Model file for the job. Use its own axes, mm. Face numbers are marked on the shaded views. A direction names the side the tool comes from. Give positions to 0.01 mm unless a question says otherwise; leave off trailing zeros. Write each loop counter-clockwise with the first axis right and the second up, starting at its lowest first coordinate (ties: lowest second). Pieces come first, ordered by that corner, then holes. Notation, with made-up numbers: (55, 74.5) - (111, 74.5) arc R30 cw to (111, 108.5) - close; hole circle Ø5 at (53.25, -3). An arc over 180 degrees is marked (long way). One line per item, written item: value. Start each with the question number.
(1) Cut at C-C, the plane z = 10. List the corners of the cut face in (x, y), and give its area (3 significant figures).
(2) Mould opens along Y. For the marked faces 1, 2, 3 and 4 say: pulls with the +Y half, pulls with the -Y half, needs draft (parallel to the pull), parting line crosses it, or undercut.
(3) Probe L1, parallel to Y at x = -2.5, z = 8; L2, parallel to Y at x = -5, z = 7; L3, parallel to X at y = -4, z = 18. List the from-to ranges inside material, lowest first.
(4) Cut at A-A, the plane x = 1.75. List the corners of the cut face in (y, z).
(5) Drop flat-ended pins along their axis: P1, Ø6, axis at y = -1, z = 6.5, coming from the -X side; P2, Ø6, axis at x = 5.5, z = 12.5, coming from the +Y side; P3, Ø8, axis at y = 3.5, z = 6, coming from the -X side. Give the stop position or say it passes through.
(6) Cut at D-D, the plane y = -8.5. List the corners of the cut face in (x, z).
(7) Cut at B-B, the plane y = 3.75. List the corners of the cut face in (x, z).
(8) 3-axis set-ups, long thin cutter, end or side, ignore diameter. For the marked faces 5 and 6: which of +Z, -Z, +X, -X, +Y, -Y reach the whole face in a straight line?
Autodesk Inventor part; units mm, degrees
ref_plane "YZ Plane" through (0, 0, 0) normal (1, 0, 0) x (0, 1, 0)
ref_plane "XZ Plane" through (0, 0, 0) normal (0, 1, 0) x (-1, 0, 0)
ref_plane "XY Plane" through (0, 0, 0) normal (0, 0, 1) x (1, 0, 0)
sketch "Sketch1" plane through (0, 0, 0) normal (0, 0, 1) x (1, 0, 0)
  line L0 (-2.6795, 10) -> (7.3205, 7.3205)
  line L1 (7.3205, 7.3205) -> (10, -2.6795)
  line L2 (10, -2.6795) -> (2.6795, -10)
  line L3 (2.6795, -10) -> (-7.3205, -7.3205)
  line L4 (-7.3205, -7.3205) -> (-10, 2.6795)
  line L5 (-10, 2.6795) -> (-2.6795, 10)
  point P0 (0, 0)
  point P1 (0, 0)
  dimension "d0" = 10
  dimension "d2" = 10
extrude "Extrusion1" add sketch "Sketch1" along normal blind 20
shell "Shell1" thickness 2 removed faces 1 at (-3.3333, 0.8932, 20)
shell "Shell2" thickness 2 removed faces 8 at (-3.3333, 0.8932, 0) at (-5.8735, 3.9776, 14) at (0.508, 7.0754, 8) at (6.3814, 3.0978, 14) at (5.8735, -3.9776, 14) at (-0.508, -7.0754, 14) at (-7.0754, -0.508, 8) at (1.8958, 1.8958, 2)
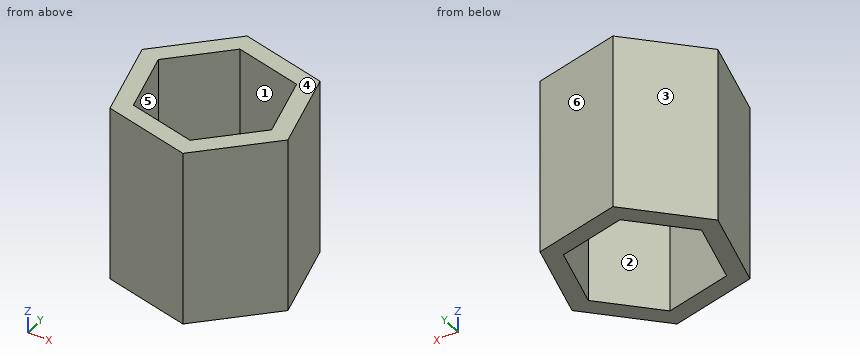
Answers follow:
1. outline: (-10, 2.68) - (-7.32, -7.32) - (2.68, -10) - (10, -2.68) - (7.32, 7.32) - (-2.68, 10) - close; hole (-7.77, 2.08) - (-5.69, -5.69) - (2.08, -7.77) - (7.77, -2.08) - (5.69, 5.69) - (-2.08, 7.77) - close
1. area: 110 mm²
2. face 1: undercut
2. face 2: undercut
2. face 3: pulls with the +Y half
2. face 4: needs draft
3. L1: y = -8.61 to -6.54, 7.35 to 9.95
3. L2: y = -7.94 to -5.87, 4.85 to 7.68
3. L3: x = -8.21 to -6.14, 5.85 to 8.68
4. outline: (-9.75, 0) - (-7.68, 0) - (-7.68, 20) - (-9.75, 20) - close; (6.74, 0) - (8.81, 0) - (8.81, 20) - (6.74, 20) - close
5. P1: stops at x = -9.82
5. P2: stops at y = 8.61
5. P3: stops at x = -10
6. outline: (-2.92, 0) - (4.18, 0) - (4.18, 20) - (-2.92, 20) - close
7. outline: (-8.93, 0) - (-6.1, 0) - (-6.1, 20) - (-8.93, 20) - close; (6.21, 0) - (8.28, 0) - (8.28, 20) - (6.21, 20) - close
8. face 5: +Z, -Z
8. face 6: +Z, -Z, +X, +Y
